Design review of the part built by this model. Coordinates are the model's own, in mm. A direction names the side the tool comes from. Round coordinates to 2 decimals unless told otherwise and drop trailing zeros. Order: outer loops, then holes, each group sorted by start corner. A loop starts at its lowest first (then second) coordinate and runs counter-clockwise, first axis right, second up. Notation, with made-up numbers: (63.5, 47.25) - (116.5, 47.25) arc R23 cw to (116.5, 66.25) - close; hole circle Ø11 at (8, 9). An arc over 180 degrees is marked (long way). Write item = value, one per line.
from build123d import *

# Parameters (mm, degrees)
F1_DEPTH = 12.7
F2_DEPTH = 6.35


with BuildPart() as f1:
    # F0 (on Front) → F1 (new body, symmetric)
    with BuildSketch(Plane.XZ):
        with BuildLine():
            ThreePointArc((-6.7687, 20.243496), (23.072752, 12.032943), (52.054703, 22.894429))
            ThreePointArc((52.054703, 22.894429), (22.847112, 31.187553), (-6.7687, 24.497039))
            ThreePointArc((-6.7687, 24.497039), (-8.459565, 23.601319), (-10.121748, 22.653433))
            ThreePointArc((-10.121748, 22.653433), (-8.470025, 21.413957), (-6.7687, 20.243496))
        make_face()
    extrude(amount=F1_DEPTH, both=True)

    # F0 (on Front) → F2 (join, symmetric)
    with BuildSketch(Plane.XZ):
        with BuildLine():
            ThreePointArc((-10.121748, 22.653433), (-8.459565, 23.601319), (-6.7687, 24.497039))
            Line((-6.7687, 24.497039), (-66.03235, 24.497039))
            Line((-66.03235, 24.497039), (-66.03235, 20.243496))
            Line((-66.03235, 20.243496), (-6.7687, 20.243496))
            ThreePointArc((-6.7687, 20.243496), (-8.470025, 21.413957), (-10.121748, 22.653433))
        make_face()
    extrude(amount=F2_DEPTH, both=True)


solid = f1.part
Item 1: For faces 1 (the face through (-36, 0, 24.497)), 2 (the face through (-8.49, -9.57, 21.43)), 3 (the face through (-37, 0, 20.243)), 4 (the face through (-8.44, 9.48, 23.61)), list the 3-axis set-ups (+Z, -Z, +X, -X, +Y, -Y) from which the entire face can be reached by the end or side of a thin tool; tool diameter is ignored.
Data:
face_1 = +Z, -X, +Y, -Y
face_2 = -Z, -X, -Y
face_3 = -Z, -X, +Y, -Y
face_4 = +Z, -X, +Y
Item 2: Take a section at A-A, the plane y = -3.25. State the section outline as (x, z) points.
Data:
outline = (-66.03, 20.24) - (-6.77, 20.24) arc R50.18 ccw to (52.05, 22.89) arc R61.5 ccw to (-6.77, 24.5) - (-66.03, 24.5) - close
Item 3: Take a section at B-B, the plane x = -44. State the section outline as (y, z) points, and give its area (3 significant figures).
Data:
outline = (-6.35, 20.24) - (6.35, 20.24) - (6.35, 24.5) - (-6.35, 24.5) - close
area = 54.0 mm2
Item 4: Insertion check: P1, Ø3, axis at y = 9, z = 16, coming from the -X side; P2, Ø10, axis at x = -50, y = -0.5, coming from the +Z side; P3, Ø1, axis at y = -7, z = 20, coming from the -X side. Each pin has a flat end and moves straight along its axis. Give the tip position at first contact, or say it passes through.
Data:
P1 = -2.06
P2 = 24.5
P3 = -7.15
Item 5: Take a section at C-C, the plane z = 13.75. State the section outline as (x, y) points.
Data:
outline = (7.61, -12.7) - (34.02, -12.7) - (34.02, 12.7) - (7.61, 12.7) - close
Item 6: For line 1 along Z through (x, y) = (-43.5, -3.75); line 2 along Y through (x, z) = (-23, 22.25); line 3 along X through (y, z) = (-2.75, 22.25), list the stretches that pass through material, from the lowest coordinate up. Write a range as [from, to].
Data:
line_1 = [20.24, 24.5]
line_2 = [-6.35, 6.35]
line_3 = [-66.03, 51.23]
